Here's how the part is built. I have some questions about the finished solid (model axes, mm). A direction names the side the tool comes from. Round coordinates to 2 decimals unless told otherwise and drop trailing zeros. Order: outer loops, then holes, each group sorted by start corner. A loop starts at its lowest first (then second) coordinate and runs counter-clockwise, first axis right, second up. Notation, with made-up numbers: (-19.5, 74) -> (14.5, 74) arc R24 ccw to (14.5, 84) -> close; hole circle Ø6 at (71.25, 23.25). An arc over 180 degrees is marked (long way). Answer in a Markdown table with one row per item.
```python
from build123d import *

# Parameters (mm, degrees)
F1_DEPTH = 20
F2_R     = 2.5
F3_DEPTH = 25
F4_R     = 5
F4_R_2   = 1.25
F5_DEPTH = 25


# Not quite as in the source:
# - a pattern or mirror of a feature is missing from the dataset's text; its kind, count and spacing are read off the source's solid


with BuildPart() as f1:
    # F0 (on Top) → F1 (new body)
    with BuildSketch(Plane.XY):
        with BuildLine():
            Line((-192, -24), (192, -24))
            Line((192, -24), (192, -9))
            Line((192, -9), (173, -9))
            ThreePointArc((173, -9), (164, 0), (173, 9))
            Line((173, 9), (192, 9))
            Line((192, 9), (192, 24))
            Line((192, 24), (-192, 24))
            Line((-192, 24), (-192, 9))
            Line((-192, 9), (-173, 9))
            ThreePointArc((-173, 9), (-164, 0), (-173, -9))
            Line((-173, -9), (-192, -9))
            Line((-192, -9), (-192, -24))
        make_face()
    extrude(amount=F1_DEPTH)

    # F2 (on face) → F3 (cut)
    with BuildSketch(Plane(origin=(-192, 0, 0), x_dir=(0, -1, 0), z_dir=(-1, 0, 0))):
        with Locations((-16, 10)):
            Circle(F2_R)
        with Locations((16, 10)):
            Circle(F2_R)
    f3 = extrude(amount=-F3_DEPTH, mode=Mode.SUBTRACT)

    # F3_copies: F3 across plane
    add(f3.mirror(Plane(origin=(0, 0, 0), x_dir=(0, 0, 1), z_dir=(1, 0, 0))), mode=Mode.SUBTRACT)

    # F4 (on face) → F5 (cut)
    with BuildSketch(Plane(origin=(0, 0, 0), x_dir=(1, 0, 0), z_dir=(0, 0, -1))):
        Circle(F4_R)
        with Locations((-5.6568542495, 5.6568542495)):
            Circle(F4_R_2)
        with Locations((-5.6568542495, -5.6568542495)):
            Circle(F4_R_2)
        with Locations((5.6568542495, -5.6568542495)):
            Circle(F4_R_2)
        with Locations((5.6568542495, 5.6568542495)):
            Circle(F4_R_2)
    extrude(amount=-F5_DEPTH, mode=Mode.SUBTRACT)


solid = f1.part
```
1. Suppose I cut it at A-A on y = 0. Write out the boundary of the cut face in (x, z).
Numbers:
| item | result |
|---|---|
| outline | (-164, 0) -> (-5, 0) -> (-5, 20) -> (-164, 20) -> close; (5, 0) -> (164, 0) -> (164, 20) -> (5, 20) -> close |
2. Suppose I cut it at B-B on z = 3. Write out the boundary of the cut face in (x, y), then the cut area to 3 significant figures.
Numbers:
| item | result |
|---|---|
| outline | (-192, -24) -> (192, -24) -> (192, -9) -> (173, -9) arc R9 cw to (173, 9) -> (192, 9) -> (192, 24) -> (-192, 24) -> (-192, 9) -> (-173, 9) arc R9 cw to (-173, -9) -> (-192, -9) -> close; hole circle Ø2.5 at (-5.66, -5.66); hole circle Ø2.5 at (-5.66, 5.66); hole circle Ø10 at (0, 0); hole circle Ø2.5 at (5.66, -5.66); hole circle Ø2.5 at (5.66, 5.66) |
| area | 17,400 mm2 |
3. We'd pull the mould along Y, two halves only. Please class faces 4 (the face through (164, 0, 10)), 5 (the face through (-3, 6, 20)), 6 (the face through (-3, -24, 10)): released by +Y, released by -Y, zero draft, split by the parting line, or undercut.
Numbers:
| item | result |
|---|---|
| face 4 | undercut |
| face 5 | zero draft |
| face 6 | released by -Y |
4. For faces 1 (the face through (-192, 18, 8)), 2 (the face through (183, -9, 10)), 3 (the face through (-183, 9, 10)), which set-ups out of +Z, -Z, +X, -X, +Y, -Y let a thin tool reach every point of the face, with its end or its side?
Numbers:
| item | result |
|---|---|
| face 1 | +Z, -Z, -X, +Y, -Y |
| face 2 | +Z, -Z, +X |
| face 3 | +Z, -Z, -X |
5. Please list where these lines run through material, in increasing order: line 1 along Z through (x, y) = (-186, 16); line 2 along X through (y, z) = (0, 6); line 3 along X through (y, z) = (-2, 14.5).
Numbers:
| item | result |
|---|---|
| line 1 | z = 0 to 7.5, 12.5 to 20 |
| line 2 | x = -164 to -5, 5 to 164 |
| line 3 | x = -164.23 to -4.58, 4.58 to 164.23 |
6. For pin 1 Ø3 at (y, z) = (-5, 9.5) entering from +X; pin 2 Ø4 at (y, z) = (-16, 10) entering from -X; pin 3 Ø4 at (y, z) = (-16, 10) entering from +X, each with a flat end and sliding along its axis, tell me the tip position at first contact or that it passes through.
Numbers:
| item | result |
|---|---|
| pin 1 | stops at x = 166.78 |
| pin 2 | stops at x = -167 |
| pin 3 | stops at x = 167 |
